Geometry check sheet. Reference: the model listing, model coordinates, mm. Face numbers are marked on the shaded views. A direction names the side the tool comes from. Give positions to 0.01 mm unless a question says otherwise; leave off trailing zeros. Loops run counter-clockwise (first coordinate to the right, second up) from the corner with the lowest first, then second, coordinate; pieces in that order, holes last. Notation, with made-up numbers: (-4.75, 84.25) - (5.25, 84.25) arc R26 ccw to (5.25, 117.25) - close; hole circle Ø5 at (26.25, 25.5). An arc over 180 degrees is marked (long way). Use a Markdown table: item, result. Add a question column.
1. Depth check by flat-ended pin: P1, Ø2, axis at x = 10.5, z = -9, coming from the +Y side; P2, Ø6, axis at y = 23, z = -25.5, coming from the +X side; P3, Ø8, axis at x = -13.5, z = -6, coming from the +Y side; P4, Ø6, axis at x = 21.5, z = 10.5, coming from the +Y side. Enter the tip coordinate at first touch or a pass-through.
2. Cross-section at A-A on z = 0. Enter the section's corners in (x, y), and give its area (3 significant figures).
3. Cross-section at B-B on y = 30. Enter the section's corners in (x, z).
4. Draft check along Z on the marked faces 3, 4 and 5. Enter one of: pulls with the +Z half, pulls with the -Z half, needs draft (parallel to the pull), parting line crosses it, or undercut.
5. Set-up check for the marked faces 1 and 2: record each of +Z, -Z, +X, -X, +Y, -Y from which the full face is reachable in a straight line by a thin tool's end or side.
6. Cross-section at C-C on x = 8. Enter the section's corners in (y, z).
7. Material ranges on L1, parallel to Z at x = -25.5, y = 30; L2, parallel to Z at x = -8, y = 30; L3, parallel to Y at x = 1, z = 20.5, recorded low to high.
8. Cross-section at D-D on x = 32. Enter the section's corners in (y, z).
from build123d import *

# Parameters (mm, degrees)
SKETCH1_W   = 75
SKETCH1_H   = 12
SKETCH1_W_2 = 40
SKETCH1_H_2 = 2


with BuildPart() as part:
    # Sketch1 → Revolve1 (revolve)
    with BuildSketch(Plane.XY):
        with Locations((0, 64)):
            Rectangle(SKETCH1_W, SKETCH1_H)
        with Locations((0, 57)):
            Rectangle(SKETCH1_W_2, SKETCH1_H_2)
    revolve(axis=Axis((-1000, 30, 0), (1, 0, 0)))


solid = part.part
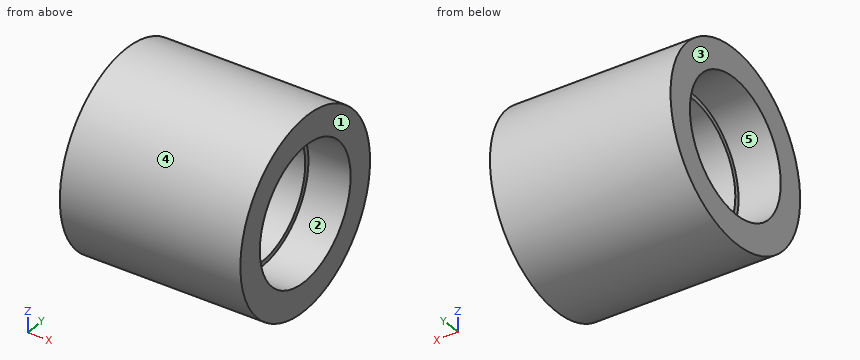
Values found:
| question | item | result |
|---|---|---|
| 1 | P1 | stops at y = 69.19 |
| 1 | P2 | stops at x = 37.5 |
| 1 | P3 | stops at y = 69.95 |
| 1 | P4 | stops at y = 69.29 |
| 2 | outline | (-37.5, -10) - (37.5, -10) - (37.5, 2) - (20, 2) - (20, 4) - (-20, 4) - (-20, 2) - (-37.5, 2) - close; (-37.5, 58) - (-20, 58) - (-20, 56) - (20, 56) - (20, 58) - (37.5, 58) - (37.5, 70) - (-37.5, 70) - close |
| 2 | area | 1,960 mm2 |
| 3 | outline | (-37.5, -40) - (37.5, -40) - (37.5, -28) - (20, -28) - (20, -26) - (-20, -26) - (-20, -28) - (-37.5, -28) - close; (-37.5, 28) - (-20, 28) - (-20, 26) - (20, 26) - (20, 28) - (37.5, 28) - (37.5, 40) - (-37.5, 40) - close |
| 4 | face 3 | needs draft |
| 4 | face 4 | parting line crosses it |
| 4 | face 5 | undercut |
| 5 | face 1 | +Z, -Z, +X, +Y, -Y |
| 5 | face 2 | +X |
| 6 | outline | circle Ø80 at (30, 0); hole circle Ø52 at (30, 0) |
| 7 | L1 | z = -40 to -28, 28 to 40 |
| 7 | L2 | z = -40 to -26, 26 to 40 |
| 7 | L3 | y = -4.35 to 14.01, 45.99 to 64.35 |
| 8 | outline | circle Ø80 at (30, 0); hole circle Ø56 at (30, 0) |
